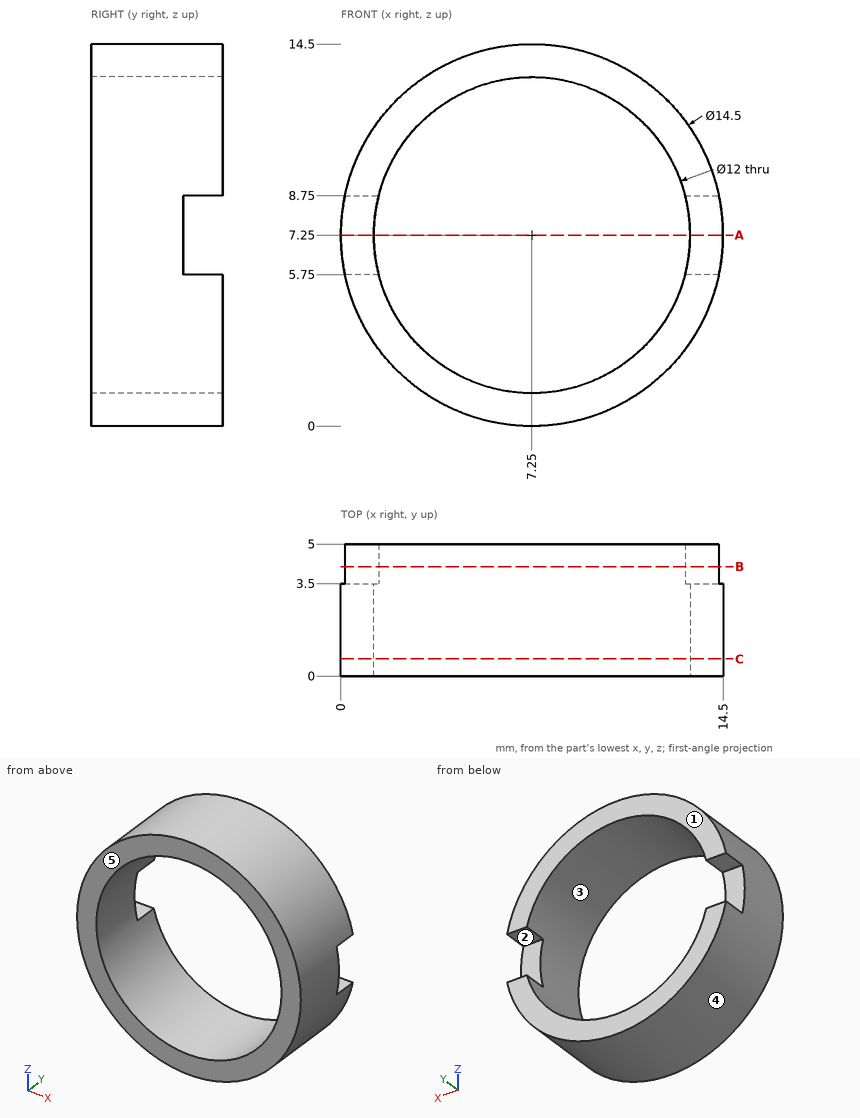
Here's the drawing with two shaded views (mm, measured from the low corner). I have some questions. A direction names the side the tool comes from. Round coordinates to 2 decimals unless told otherwise and drop trailing zeros. Loops run counter-clockwise (first coordinate to the right, second up) from the corner with the lowest first, then second, coordinate; pieces in that order, holes last.
1. If I drill on probe 1 along X at (y, z) = (3.1, 7.25); probe 2 along Z at (x, y) = (8.5, 3.4), over which ranges is the centre line in solid material (lowest first)?
Answers:
probe 1: x = 0 to 1.25, 13.25 to 14.5
probe 2: z = 0.11 to 1.38, 13.12 to 14.39
2. Suppose I cut it at B-B, the plane y = 4.15. Please give me the cut outline in (x, z), and give its area (3 significant figures).
Answers:
outline: (0.16, 5.75) arc R7.25 ccw to (14.34, 5.75) - (13.06, 5.75) arc R6 cw to (1.44, 5.75) - close; (0.16, 8.75) - (1.44, 8.75) arc R6 cw to (13.06, 8.75) - (14.34, 8.75) arc R7.25 ccw to start
area: 44.5 mm2
3. Will these pins go through, and if not, where does the flat tip stop? pin 1 (1 mm diameter, centred on x = 9.5, y = 4, fed in from +Z); pin 2 (1.4 mm diameter, centred on x = 1, y = 4, fed in from +Z); pin 3 (0.7 mm diameter, centred on x = 14, z = 6.5, fed in from +Y).
Answers:
pin 1: stops at z = 14.29
pin 2: stops at z = 11.91
pin 3: stops at y = 3.5
4. Thinking about a two-plate mould opening in Z: for the marked faces 3, 4 and 5, which applies, released by +Z, released by -Z, zero draft, split by the parting line, or undercut?
Answers:
face 3: undercut
face 4: split by the parting line
face 5: zero draft
5. For the marked faces 1 and 2, which set-ups out of +Z, -Z, +X, -X, +Y, -Y let a thin tool reach every point of the face, with its end or its side?
Answers:
face 1: +Z, -Z, +X, -X, +Y
face 2: +X, -X, +Y
6. Suppose I cut it at C-C, the plane y = 0.65. Please give me the cut outline in (x, z), and give its area (3 significant figures).
Answers:
outline: circle Ø14.5 at (7.25, 7.25); hole circle Ø12 at (7.25, 7.25)
area: 52.0 mm2
7. Suppose I cut it at A-A, the plane z = 7.25. Please give me the cut outline in (x, y).
Answers:
outline: (0, 0) - (1.25, 0) - (1.25, 3.5) - (0, 3.5) - close; (13.25, 0) - (14.5, 0) - (14.5, 3.5) - (13.25, 3.5) - close
